Part print with two shaded views. Sizes in mm from the minimum x, y, z corner. A direction names the side the tool comes from. Round coordinates to 2 decimals unless told otherwise and drop trailing zeros. Write each loop counter-clockwise with the first axis right and the second up, starting at its lowest first coordinate (ties: lowest second). Pieces come first, ordered by that corner, then holes. Notation, with made-up numbers: M 57,-0.75 L 109,-0.75 A23 cw 109,20.25 Z; hole C 48.5,10 d1. An arc over 180 degrees is marked long. One line per question, with ' | ' between items. Start each with the question number.
1) Tool access for the marked faces 1 and 2: list every direction of +Z, -Z, +X, -X, +Y, -Y with a clear straight run to the whole face (end or side of a thin tool).
2) Drop flat-ended pins along their axis: pin 1 Ø1.8 at (x, z) = (4, 9) entering from +Y; pin 2 Ø3 at (x, y) = (3, 59) entering from -Z. Give the stop position or say it passes through.
3) Wall check: probe 1 along Z at (x, y) = (5.4, 80.5); probe 2 along Z at (x, y) = (4.3, 57); probe 3 along Y at (x, z) = (1.25, 8). Give the ranges that are in metal, low to high. Write a range as [from, to].
4) Saw through at D-D (z = 10.5). List the corners of the cut face in (x, y), plus the area to 3 significant figures.
5) Saw through at B-B (y = 98). List the corners of the cut face in (x, z), plus the area to 3 significant figures.
6) Saw through at C-C (x = 1.7). List the corners of the cut face in (y, z).
7) Saw through at A-A (z = 4.5). List the corners of the cut face in (x, y), plus the area to 3 significant figures.
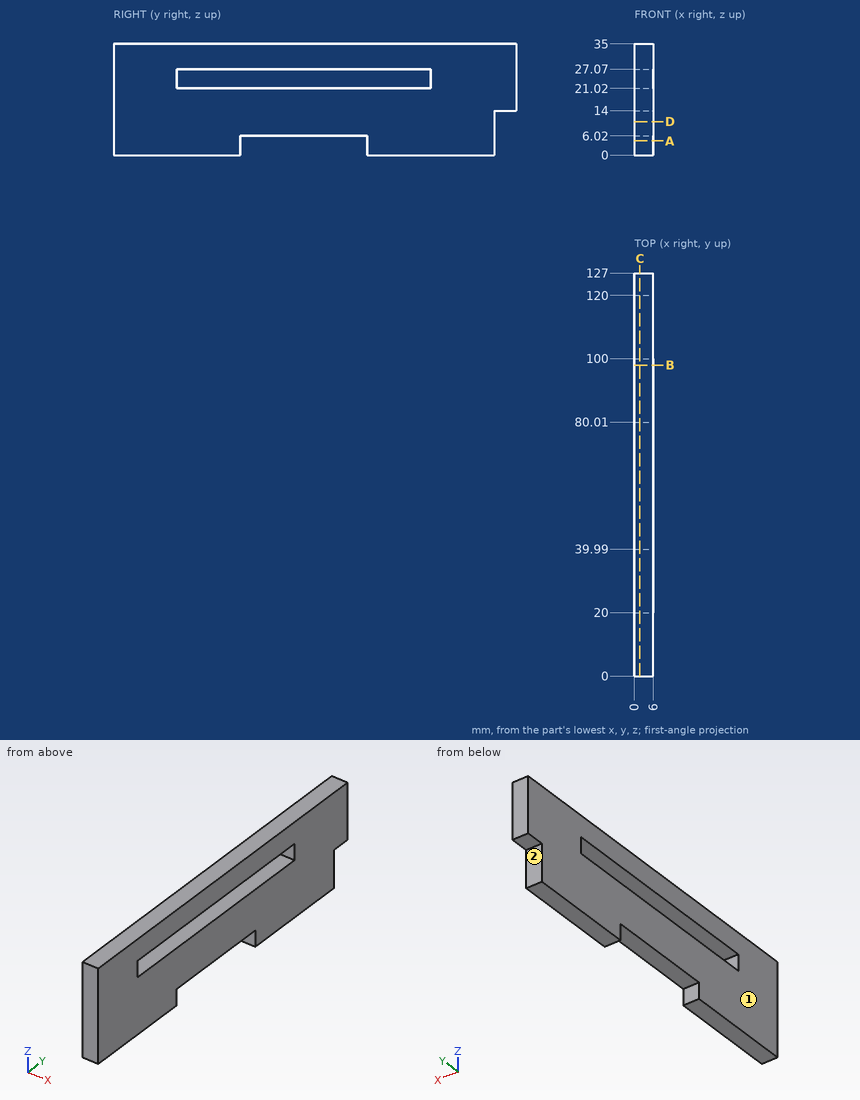
Answer key:
1) face 1: +Z, -Z, -X, +Y, -Y | face 2: -Z, +X, -X, +Y
2) pin 1: stops at y = 120 | pin 2: stops at z = 6.02
3) probe 1: z = [0, 21.02], [27.07, 35] | probe 2: z = [6.02, 21.02], [27.07, 35] | probe 3: y = [0, 120]
4) outline: M 0,0 L 6,0 L 6,120 L 0,120 Z | area: 720 mm2
5) outline: M 0,0 L 6,0 L 6,21.02 L 0,21.02 Z; M 0,27.07 L 6,27.07 L 6,35 L 0,35 Z | area: 174 mm2
6) outline: M 0,0 L 39.99,0 L 39.99,6.02 L 80.01,6.02 L 80.01,0 L 120,0 L 120,14 L 127,14 L 127,35 L 0,35 Z; hole M 20,21.02 L 100,21.02 L 100,27.07 L 20,27.07 Z
7) outline: M 0,0 L 6,0 L 6,39.99 L 0,39.99 Z; M 0,80.01 L 6,80.01 L 6,120 L 0,120 Z | area: 480 mm2
